from build123d import *

# Parameters (mm, degrees)
EXTRUDE_1_DEPTH     = 28.9
CHAMFER_1_SIZE      = 0.5
CUT_EXTRUDE_1_DEPTH = 0.3
SKETCH_6_W          = 0.2
SKETCH_6_H          = 4.8
CUT_EXTRUDE_2_DEPTH = 8.3
CHAMFER_2_SIZE      = 1
CHAMFER_3_SIZE      = 0.6
CHAMFER_4_SIZE      = 0.5
SKETCH_7_R          = 0.4
CUT_EXTRUDE_3_DEPTH = 19.3


with BuildPart() as part:
    # 草图1 → 凸台-拉伸1 (new body)
    with BuildSketch(Plane.XY):
        Polygon((-10, 0), (-10, 8), (10, 8), (10, 0), (4.5, 0), (4.5, 1), (4.146446609, 1.353553391), (3.646446609, 1.353553391), (3.646446609, 1.853553391), (4.146446609, 1.853553391), (4.5, 2.207106781), (4.5, 4.5), (-4.5, 4.5), (-4.5, 2.207106781), (-4.146446609, 1.853553391), (-3.646446609, 1.853553391), (-3.646446609, 1.353553391), (-4.146446609, 1.353553391), (-4.5, 1), (-4.5, 0), align=None)
    extrude(amount=-EXTRUDE_1_DEPTH)

    # 草图3 → M3 螺纹孔1 (revolve, cut)
    with BuildSketch(Plane(origin=(7.5, 8, -19.45), x_dir=(0, 0, 1), z_dir=(1, 0, 0))):
        Polygon((0, 0), (0, 3.751075774), (1.25, 3), (1.25, 0), align=None)
    hole_wizard_m3_1 = revolve(axis=Axis((7.5, 14.35, -19.45), (0, -1, 0)), mode=Mode.SUBTRACT)

    # 镜向1: M3 螺纹孔1 across plane
    add(hole_wizard_m3_1.mirror(Plane(origin=(0, 0, -14.45), x_dir=(1, 0, 0), z_dir=(0, 0, -1))), mode=Mode.SUBTRACT)

    # 镜向2: M3 螺纹孔1 across plane
    add(hole_wizard_m3_1.mirror(Plane.ZY), mode=Mode.SUBTRACT)

    # 镜向2 copy 1 sketch → 镜向2 copy 1 (revolve, cut)
    with BuildSketch(Plane(origin=(-7.5, 8, -9.45), x_dir=(0, 0, -1), z_dir=(-1, 0, 0))):
        Polygon((0, 0), (0, 3.751075774), (1.25, 3), (1.25, 0), align=None)
    revolve(axis=Axis((-7.5, 14.35, -9.45), (0, -1, 0)), mode=Mode.SUBTRACT)

    # 倒角1
    chamfer_1_edges = [part.edges().sort_by_distance(p)[0] for p in [
        (10, 8, -14.45),
        (-10, 8, -14.45),
    ]]
    chamfer(chamfer_1_edges, length=CHAMFER_1_SIZE)

    # 草图5 → 切除-拉伸1 (cut)
    with BuildSketch(Plane(origin=(0, 8, 0), x_dir=(1, 0, 0), z_dir=(0, 1, 0))):
        Polygon((-9.5, 24.1), (-4.368581018, 24.1), (-4.368581018, 4.8), (-9.5, 4.8), (-10, 4.8), (-10, 0), (10, 0), (10, 4.8), (9.5, 4.8), (4.368581018, 4.8), (4.368581018, 24.1), (9.5, 24.1), (10, 24.1), (10, 28.9), (-10, 28.9), (-10, 24.1), align=None)
    extrude(amount=-CUT_EXTRUDE_1_DEPTH, mode=Mode.SUBTRACT)

    # 草图6 → 切除-拉伸2 (cut)
    with BuildSketch(Plane(origin=(0, 7.7, 0), x_dir=(1, 0, 0), z_dir=(0, 1, 0))):
        with Locations((-9.9, 26.5)):
            Rectangle(SKETCH_6_W, SKETCH_6_H)
        with Locations((9.9, 26.5)):
            Rectangle(SKETCH_6_W, SKETCH_6_H)
        with Locations((9.9, 2.4)):
            Rectangle(SKETCH_6_W, SKETCH_6_H)
        with Locations((-9.9, 2.4)):
            Rectangle(SKETCH_6_W, SKETCH_6_H)
    extrude(amount=-CUT_EXTRUDE_2_DEPTH, mode=Mode.SUBTRACT)

    # 倒角2
    # the kernel refuses this chamfer: 1 mm, written as the material it takes off along each edge
    with BuildSketch(Plane(origin=(-9.8, 7.7, -4.8), x_dir=(-0.027495876610583895, -0.9996219169112968, 0), z_dir=(0, 0, 1)), Plane(origin=(-9.8, 7.7, -31.471682988), x_dir=(-0.027495876610585623, -0.9996219169112968, 0), z_dir=(0, 0, 1))) as chamfer_2_piece_1:
        Polygon((CHAMFER_2_SIZE * 0.999621916911, CHAMFER_2_SIZE * 0.0274958766106), (-CHAMFER_2_SIZE * 0.0274958766106, CHAMFER_2_SIZE * 0.999621916911), (0, 0), align=None)
    extrude(amount=7.371682988, mode=Mode.SUBTRACT)
    with BuildSketch(Plane(origin=(9.8, 7.7, 2.571682988), x_dir=(-0.9996219169112968, 0.02749587661058651, 0), z_dir=(0, 0, -1)), Plane(origin=(9.8, 7.7, -24.1), x_dir=(-0.9996219169112968, 0.02749587661058651, 0), z_dir=(0, 0, -1))) as chamfer_2_piece_2:
        Polygon((CHAMFER_2_SIZE * 0.999621916911, -CHAMFER_2_SIZE * 0.0274958766106), (-CHAMFER_2_SIZE * 0.0274958766106, -CHAMFER_2_SIZE * 0.999621916911), (0, 0), align=None)
    extrude(amount=7.371682988, mode=Mode.SUBTRACT)

    # 倒角3
    chamfer_3_edges = [part.edges().sort_by_distance(p)[0] for p in [
        (-9.8, 0, -26.5),
        (9.8, 0, -26.5),
        (9.8, 0, -2.4),
        (-9.8, 0, -2.4),
    ]]
    chamfer(chamfer_3_edges, length=CHAMFER_3_SIZE)

    # 倒角4
    chamfer_4_edges = [part.edges().sort_by_distance(p)[0] for p in [
        (-10, 0, -14.45),
        (10, 0, -14.45),
    ]]
    chamfer(chamfer_4_edges, length=CHAMFER_4_SIZE)

    # 草图7 → 切除-拉伸3 (cut)
    with BuildSketch(Plane(origin=(0, 0, -24.1), x_dir=(-1, 0, 0), z_dir=(0, 0, -1))):
        with Locations((-10.2, 4)):
            Circle(SKETCH_7_R)
    extrude(amount=-CUT_EXTRUDE_3_DEPTH, mode=Mode.SUBTRACT)


solid = part.part
The listing builds one solid part. Answer for the finished solid, in the listing's coordinates (mm). A direction names the side the tool comes from. Coordinates: 2 decimals unless noted, no trailing zeros. Order: outer loops, then holes, each group sorted by start corner. A loop starts at its lowest first (then second) coordinate and runs counter-clockwise, first axis right, second up.
Q1. A cutting plane is placed at D-D, the plane x = -1.25. Write down the section's boundary in (y, z).
Q2. A cutting plane is placed at C-C, the plane y = 6.25. Write down the section's boundary in (x, z).
Q3. Consider line 1 (X direction, y = 6.25, z = -9.45); line 2 (Z direction, x = 7.5, y = 6.5); line 3 (Y direction, x = -4, z = -15.25). Determine where each line is inside the solid, lowest interval first.
Q4. A cutting plane is placed at A-A, the plane y = 3.25. Write down the section's boundary in (x, z).
Q5. Given P1, Ø2.5, axis at y = 4.5, z = -1.5, coming from the -X side; P2, Ø5, axis at x = 0.5, z = -25, coming from the -Y side; P3, Ø2.5, axis at y = 2.5, z = -3, coming from the +X side, each flat-ended and moving along its own axis, determine where each tip first touches the part or whether it passes through.
Q6. For a pull along Y with two mould halves and no side action, classify faces 5 (the face through (4.5, 0.5, -14.2)), 6 (the face through (-7, 0, -14)), 7 (the face through (-4.5, 3, -14)) as pulls with the +Y half, pulls with the -Y half, needs draft (parallel to the pull), parting line crosses it, or undercut.
Q7. Which of the six approach directions +Z, -Z, +X, -X, +Y, -Y give full straight-line access (tool end or side, diameter ignored) to faces 1 (the face through (-9.3, 7.2, -26.5)), 2 (the face through (-4.5, 0.5, -14.2)), 3 (the face through (9.8, 4, -2)), 4 (the face through (9.8, 4, -26))?
Answers follow:
1. outline: (4.5, -28.9) - (7.7, -28.9) - (7.7, 0) - (4.5, 0) - close
2. outline: (-10, -24.1) - (-9.8, -24.1) - (-9.8, -28.9) - (9.8, -28.9) - (9.8, -24.1) - (10, -24.1) - (10, -4.8) - (9.8, -4.8) - (9.8, 0) - (-9.8, 0) - (-9.8, -4.8) - (-10, -4.8) - close; hole circle Ø2.5 at (-7.5, -19.45); hole circle Ø2.5 at (-7.5, -9.45); hole circle Ø2.5 at (7.5, -19.45); hole circle Ø2.5 at (7.5, -9.45)
3. line 1: x = -10 to -8.75, -6.25 to 6.25, 8.75 to 10
3. line 2: z = -28.9 to -20.7, -18.2 to -10.7, -8.2 to 0
3. line 3: y = 1.35 to 1.85, 4.5 to 7.7
4. outline: (-10, -24.1) - (-9.8, -24.1) - (-9.8, -28.9) - (-4.5, -28.9) - (-4.5, 0) - (-9.8, 0) - (-9.8, -4.8) - (-10, -4.8) - close; (4.5, -28.9) - (9.8, -28.9) - (9.8, -24.1) - (10, -24.1) - (10, -4.8) - (9.8, -4.8) - (9.8, 0) - (4.5, 0) - close
5. P1: stops at x = -9.8
5. P2: stops at y = 4.5
5. P3: stops at x = 9.8
6. face 5: needs draft
6. face 6: pulls with the -Y half
6. face 7: undercut
7. face 1: -Z, -X, +Y
7. face 2: +Z, -Z, -Y
7. face 3: +Z, +X, +Y, -Y
7. face 4: -Z, +X, +Y, -Y
